Here's how the part is built. I have some questions about the finished solid (model axes, mm). Face numbers are marked on the shaded views. Round coordinates to 2 decimals unless told otherwise and drop trailing zeros. Loops run counter-clockwise (first coordinate to the right, second up) from the corner with the lowest first, then second, coordinate; pieces in that order, holes last. Notation, with made-up numbers: M -2.5,29 L 1.5,29 A18 ccw 1.5,52 Z; hole C 5,-39 d4. An arc over 180 degrees is marked long. Answer as a JSON object with one key per item and string values.
Autodesk Inventor part; units mm, degrees
ref_plane "YZ Plane" through (0, 0, 0) normal (1, 0, 0) x (0, 1, 0)
ref_plane "XZ Plane" through (0, 0, 0) normal (0, 1, 0) x (-1, 0, 0)
ref_plane "XY Plane" through (0, 0, 0) normal (0, 0, 1) x (1, 0, 0)
sketch "Sketch1" plane through (0, 0, 0) normal (0, 0, 1) x (1, 0, 0)
  line L0 (0, 0) -> (69.215, 0)
  line L1 (69.215, 0) -> (69.215, -103.124)
  line L2 (69.215, -103.124) -> (0, -103.124)
  line L3 (0, -103.124) -> (0, 0)
  dimension "d0" = 69.215
  dimension "d1" = 103.124
extrude "Extrusion1" add sketch "Sketch1" along normal blind 22.225
fillet "Fillet1" radius 4.445 3 edges at (0, 0, 11.1125) (69.215, 0, 11.1125) (0, -103.124, 11.1125)
fillet "Fillet2" radius 4.445 1 edges at (69.215, -103.124, 11.1125)
sketch "Sketch2" plane through (0, -98.679, 0) normal (-1, 0, 0) x (0, 0, 1)
  line L0 (0, 0) -> (0, 94.234)
  line L1 (22.225, 94.234) -> (0, 94.234)
  line L2 (0, 98.679) -> (22.225, 98.679)
  line L3 (5.461, 94.234) -> (18.161, 94.234)
  line L4 (18.161, 94.234) -> (18.161, 14.859)
  line L5 (18.161, 14.859) -> (5.461, 14.859)
  line L6 (5.461, 14.859) -> (5.461, 94.234)
  dimension "d8" = 12.7
  dimension "d9" = 79.375
extrude "Extrusion2" cut sketch "Sketch2" against normal blind 12.7
sketch "Sketch3" plane through (0, 0, 22.225) normal (0, 0, 1) x (1, 0, 0)
  line L0 (64.77, 0) -> (4.445, 0)
  circle A0 centre (33.02, -22.86) radius 0.635
  point P0 (0, 0)
extrude "Extrusion3" cut sketch "Sketch3" against normal blind 12.7
properties part number "Ethernet switch" material "Acetal Resin, White"
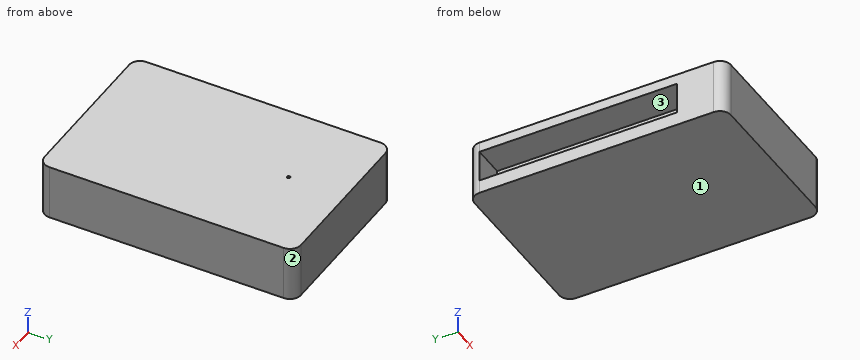
Item 1: We'd pull the mould along Y, two halves only. Please class the marked faces 1, 2 and 3: +Y half, -Y half, draft (parallel to the pull), parting line (faces both ways), or undercut.
Solution:
{"face 1": "draft", "face 2": "+Y half", "face 3": "undercut"}
Item 2: I want a section at A-A on x = 8. List the corners of the cut face in (y, z) for me (3 decimals), plus the area to 3 significant figures.
Solution:
{"outline": "M -103.124,0 L 0,0 L 0,22.225 L -103.124,22.225 Z; hole M -83.82,5.461 L -4.445,5.461 L -4.445,18.161 L -83.82,18.161 Z", "area": "1,280 mm2"}
Item 3: I want a section at B-B on z = 15.75. List the corners of the cut face in (x, y) for me (3 decimals).
Solution:
{"outline": "M 0,-98.679 A4.445 ccw 4.445,-103.124 L 64.77,-103.124 A4.445 ccw 69.215,-98.679 L 69.215,-4.445 A4.445 ccw 64.77,0 L 4.445,0 A4.445 ccw 0,-4.445 L 12.7,-4.445 L 12.7,-83.82 L 0,-83.82 Z; hole C 33.02,-22.86 d1.27"}
Item 4: I want a section at C-C on y = -81. List the corners of the cut face in (x, z) for me (3 decimals).
Solution:
{"outline": "M 0,0 L 69.215,0 L 69.215,22.225 L 0,22.225 L 0,18.161 L 12.7,18.161 L 12.7,5.461 L 0,5.461 Z"}
Item 5: If I drill on L1, parallel to Y at x = 33.02, z = 16.5 (3 decimals); L2, parallel to Z at x = 8.5, y = -75.5 (3 decimals); L3, parallel to X at y = -23, z = 15.25 (3 decimals), over which ranges is the centre line in solid material (lowest first)? Write a range as from..to.
Solution:
{"L1": "y = -103.124..-23.495, -22.225..0", "L2": "z = 0..5.461, 18.161..22.225", "L3": "x = 12.7..32.401, 33.639..69.215"}
Item 6: For P1, Ø10, axis at x = 3.5, z = 13.5, coming from the +Y side; P2, Ø6.5, axis at y = -32.5, z = 9, coming from the -X side, each with a flat end and sliding along its axis, tell me the tip position at first contact or that it passes through.
Solution:
{"P1": "stops at y = 0", "P2": "stops at x = 12.7"}
